Geometry: final body of the model. Coordinates: model frame, mm. Round coordinates to 2 decimals unless told otherwise and drop trailing zeros. Order: outer loops, then holes, each group sorted by start corner. A loop starts at its lowest first (then second) coordinate and runs counter-clockwise, first axis right, second up. Notation, with made-up numbers: M 6.25,3 L 44.25,3 A6 cw 44.25,13 Z; hole C 53.25,-39.75 d11. An arc over 180 degrees is marked long. Return JSON: item names as keys, results as strings. Group by question number.
Q1. Cut plane A-A on x = 12. Output: boundary loops of the cut face in (y, z), and give its area (3 significant figures).
Q2. Ray query, probe 1 along Y at (x, z) = (12.5, -309); probe 2 along Z at (x, y) = (15, 55.5). Return the intervals inside material, ascending.
Q3. Contact query for a flat-ended pin moving along its axis: pin 1 (7 mm diameter, centred on x = 11.5, z = -2.5, fed in from +Y). Output: stop coordinate, or through.
Q4. Mould query, pull axis Z, two halves, no side actions, for faces 1 (the face through (8, 119, 0)), 2 (the face through (0, 129, -219)), 3 (the face through (9.525, 126, -26)), 4 (the face through (8, 125, -444.5)). Classes: released by +Z, released by -Z, zero draft, split by the parting line, or undercut.
```python
from build123d import *

# Parameters (mm, degrees)
BOSS_EXTRUDE1_DEPTH = 15.875
SKETCH2_W           = 6.35
SKETCH2_H           = 6.35
CUT_EXTRUDE1_DEPTH  = 445.5
CUT_EXTRUDE3_REACH  = 256
SKETCH3_W           = 6.35
SKETCH3_H           = 6.35
CUT_EXTRUDE4_REACH  = 256
SKETCH4_W           = 6.35
SKETCH4_H           = 6.35


with BuildPart() as part:
    # Sketch1 → Boss-Extrude1 (new body)
    with BuildSketch(Plane(origin=(0, 0, 0), x_dir=(0, 0, -1), z_dir=(1, 0, 0))):
        with BuildLine():
            Line((0, 0), (444.5, 0))
            Line((444.5, 0), (444.5, 254))
            Line((444.5, 254), (19.05, 254))
            ThreePointArc((19.05, 254), (5.579615818, 248.420384182), (0, 234.95))
            Line((0, 234.95), (0, 0))
        make_face()
    extrude(amount=BOSS_EXTRUDE1_DEPTH)

    # Sketch2 → Cut-Extrude1 (cut, through all)
    with BuildSketch(Plane(origin=(0, 0, -444.5), x_dir=(-1, 0, 0), z_dir=(0, 0, -1))):
        with Locations((-12.7, 47.625)):
            Rectangle(SKETCH2_W, SKETCH2_H)
    extrude(amount=-CUT_EXTRUDE1_DEPTH, mode=Mode.SUBTRACT)

    # Sketch3 → Cut-Extrude3 (cut, up to next)
    with BuildSketch(Plane.XZ, mode=Mode.PRIVATE) as cut_extrude3_sk1:
        with Locations((12.7, -9.525)):
            Rectangle(SKETCH3_W, SKETCH3_H)
    cut_extrude3_tool1 = extrude(cut_extrude3_sk1.sketch, amount=-CUT_EXTRUDE3_REACH, mode=Mode.PRIVATE) & part.part
    add(cut_extrude3_tool1.solids().sort_by_distance((12.7, 0, -9.525))[0], mode=Mode.SUBTRACT)

    # Sketch4 → Cut-Extrude4 (cut, up to next)
    with BuildSketch(Plane(origin=(0, 254, 0), x_dir=(1, 0, 0), z_dir=(0, 1, 0)), mode=Mode.PRIVATE) as cut_extrude4_sk1:
        with Locations((12.7, 28.575)):
            Rectangle(SKETCH4_W, SKETCH4_H)
    cut_extrude4_tool1 = extrude(cut_extrude4_sk1.sketch, amount=-CUT_EXTRUDE4_REACH, mode=Mode.PRIVATE) & part.part
    add(cut_extrude4_tool1.solids().sort_by_distance((12.7, 254, -28.575))[0], mode=Mode.SUBTRACT)


solid = part.part
```
Result sheet:
{
 "1": {"outline": "M 0,-444.5 L 44.45,-444.5 L 44.45,-12.7 L 0,-12.7 Z; M 0,-6.35 L 44.45,-6.35 L 44.45,0 L 0,0 Z; M 50.8,-444.5 L 254,-444.5 L 254,-31.75 L 50.8,-31.75 Z; M 50.8,-25.4 L 254,-25.4 L 254,-19.05 A19.05 ccw 234.95,0 L 50.8,0 Z", "area": "108,000 mm²"},
 "2": {"probe 1": "y = 0 to 44.45, 50.8 to 254", "probe 2": "z = -444.5 to -31.75, -25.4 to 0"},
 "3": {"pin 1": "stops at y = 248.83"},
 "4": {"face 1": "released by +Z", "face 2": "zero draft", "face 3": "undercut", "face 4": "released by -Z"}
}
